Verification items for the finished model (mm, model axes). Face numbers are marked on the shaded views. A direction names the side the tool comes from. Coordinates: 2 decimals unless noted, no trailing zeros. Write each loop counter-clockwise with the first axis right and the second up, starting at its lowest first coordinate (ties: lowest second). Pieces come first, ordered by that corner, then holes. Notation, with made-up numbers: (88, -36.75) -> (94, -36.75) arc R16 cw to (94, -6.75) -> close; hole circle Ø5 at (84, 36). An arc over 180 degrees is marked (long way). Write each question's results on one line, items separated by ' | '. Start each with the question number.
from build123d import *

# Parameters (mm, degrees)
SKETCH_W        = 64.8
SKETCH_H        = 40
PAD_DEPTH       = 40
POCKET_DEPTH    = 64.801
POCKET001_DEPTH = 64.801
POCKET002_DEPTH = 64.801
SKETCH004_W     = 60.8
SKETCH004_H     = 10.4
POCKET003_DEPTH = 30
POCKET004_DEPTH = 15.5651335663
POCKET005_DEPTH = 64.801


with BuildPart() as part:
    # Sketch → Pad (new body)
    with BuildSketch(Plane.XY):
        with Locations((32.4, 20)):
            Rectangle(SKETCH_W, SKETCH_H)
    extrude(amount=PAD_DEPTH)

    # Sketch001 → Pocket (cut, through all)
    with BuildSketch(Plane.YZ.offset(64.8)):
        Polygon((0, 0), (0, 40), (14.5588093668, 40), align=None)
    extrude(amount=-POCKET_DEPTH, mode=Mode.SUBTRACT)

    # Sketch002 → Pocket001 (cut, through all)
    with BuildSketch(Plane.YZ.offset(64.8)):
        Polygon((29.7588093668, 40), (18.8397023417, 10), (40, 10), (40, 40), align=None)
    extrude(amount=-POCKET001_DEPTH, mode=Mode.SUBTRACT)

    # Sketch003 → Pocket002 (cut, through all)
    with BuildSketch(Plane.YZ.offset(64.8)):
        Polygon((14.5588093668, 40), (27.9807471354, 35.1148141674), (29.7588093668, 40), align=None)
    extrude(amount=-POCKET002_DEPTH, mode=Mode.SUBTRACT)

    # Sketch004 → Pocket003 (cut)
    with BuildSketch(Plane(origin=(0, 14.5588093668, 40), x_dir=(1, 0, 0), z_dir=(0, 0.3420201432, 0.9396926208))):
        with Locations((32.4, 7.0833278364)):
            Rectangle(SKETCH004_W, SKETCH004_H)
    extrude(amount=-POCKET003_DEPTH, mode=Mode.SUBTRACT)

    # Sketch005 → Pocket004 (cut, through all)
    with BuildSketch(Plane(origin=(0, 1.7697492704, -0.6441360564), x_dir=(-1, 0, 0), z_dir=(0, 0.9396926208, -0.3420201432))):
        Polygon((-39.795, 21.5671108977), (-39.795, 12.5671108977), (-24.795, 12.5671108977), (-24.795, 21.5671108977), (-4, 21.5671108977), (-4, 42.5671108977), (-60.8, 42.5671108977), (-60.59, 21.5671108977), align=None)
    extrude(amount=-POCKET004_DEPTH, mode=Mode.SUBTRACT)

    # Sketch006 → Pocket005 (cut, through all)
    with BuildSketch(Plane.YZ.offset(64.8)):
        Polygon((27.9807471354, 35.1148141674), (12.7807471354, 35.1148141674), (14.5588093668, 40), align=None)
    extrude(amount=-POCKET005_DEPTH, mode=Mode.SUBTRACT)


solid = part.part
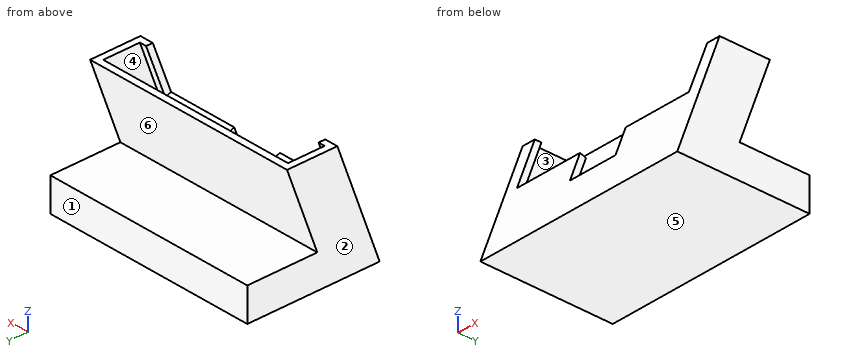
1. Sectioned sample at D-D on y = 10.5. Record the cut outline in (x, z), plus the area to 3 significant figures.
2. Sectioned sample at A-A on y = 25. Record the cut outline in (x, z), plus the area to 3 significant figures.
3. Mould release check, pull along X, two halves, no side actions. Record for the marked faces 1, 2 and 3: +X half, -X half, draft (parallel to the pull), parting line (faces both ways), or undercut.
4. Depth check by flat-ended pin: pin 1 Ø10 at (x, z) = (29, 7.5) entering from -Y; pin 2 Ø1 at (x, z) = (49, 30) entering from +Y; pin 3 Ø6 at (x, y) = (22.5, 32) entering from +Z. Enter the tip coordinate at first touch or a pass-through.
5. Sectioned sample at C-C on z = 24. Record the cut outline in (x, y).
6. Material ranges on probe 1 along X at (y, z) = (16.5, 34); probe 2 along Z at (x, y) = (7.5, 36.5); probe 3 along Y at (x, z) = (7, 18), recorded low to high. Write a range as from..to.
7. Sectioned sample at B-B on x = 10. Record the cut outline in (y, z), plus the area to 3 significant figures.
8. Tool access check on the marked faces 4, 5 and 6. Record the directions out of +Z, -Z, +X, -X, +Y, -Y that give a thin tool (end or side, any length) a straight path to the whole face; none if there is none.
Computed values:
1) outline: (0, 0) -> (64.8, 0) -> (64.8, 28.85) -> (60.68, 28.85) -> (60.63, 23.34) -> (62.8, 23.34) -> (62.8, 9.55) -> (2, 9.55) -> (2, 23.34) -> (4, 23.34) -> (4, 28.85) -> (0, 28.85) -> close | area: 719 mm^2
2) outline: (0, 0) -> (64.8, 0) -> (64.8, 10) -> (0, 10) -> close; (0, 26.93) -> (64.8, 26.93) -> (64.8, 35.11) -> (62.8, 35.11) -> (62.8, 32.77) -> (2, 32.77) -> (2, 35.11) -> (0, 35.11) -> close | area: 1,040 mm^2
3) face 1: draft | face 2: -X half | face 3: undercut
4) pin 1: stops at y = 0.91 | pin 2: stops at y = 26.3 | pin 3: stops at z = 10
5) outline: (0, 8.74) -> (4, 8.74) -> (4, 10.74) -> (2, 10.74) -> (2, 21.81) -> (62.8, 21.81) -> (62.8, 10.74) -> (60.64, 10.74) -> (60.63, 8.74) -> (64.8, 8.74) -> (64.8, 23.94) -> (0, 23.94) -> close
6) probe 1: x = 0..2, 62.8..64.8 | probe 2: z = 0..10 | probe 3: y = 6.55..8.56, 19.62..21.75
7) outline: (0, 0) -> (40, 0) -> (40, 10) -> (18.84, 10) -> (27.98, 35.11) -> (25.85, 35.11) -> (15.84, 7.61) -> (6.07, 11.17) -> (9.15, 19.62) -> (7.38, 20.27) -> close | area: 448 mm^2
8) face 4: none | face 5: -Z, +X, -X, +Y, -Y | face 6: +X, -X, +Y
